```python
from build123d import *

# Parameters (mm, degrees)
SKETCH1_R           = 6
BOSS_EXTRUDE1_DEPTH = 44
SKETCH2_W           = 88
SKETCH2_H           = 20
CUT_EXTRUDE1_DEPTH  = 159.811208672
FILLET1_R           = 5


with BuildPart() as part:
    # Sketch1 → Boss-Extrude1 (new body)
    with BuildSketch(Plane.XY):
        with BuildLine():
            Line((0, 11), (140, 11))
            ThreePointArc((140, 11), (151, 0), (140, -11))
            Line((140, -11), (0, -11))
            ThreePointArc((0, -11), (-11, 0), (0, 11))
        make_face()
        Circle(SKETCH1_R, mode=Mode.SUBTRACT)
        with Locations((140, 0)):
            Circle(SKETCH1_R, mode=Mode.SUBTRACT)
    extrude(amount=BOSS_EXTRUDE1_DEPTH)

    # Sketch2 → Cut-Extrude1 (cut, through all)
    with BuildSketch(Plane(origin=(0, 11, 0), x_dir=(1, 0, 0), z_dir=(0, 1, 0))):
        with Locations((-11, -22)):
            Rectangle(SKETCH2_W, SKETCH2_H)
    extrude(amount=-CUT_EXTRUDE1_DEPTH, mode=Mode.SUBTRACT)

    # Fillet1
    fillet1_edges = [part.edges().sort_by_distance(p)[0] for p in [
        (33, 0, 32),
        (33, 0, 12),
    ]]
    fillet(fillet1_edges, radius=FILLET1_R)


solid = part.part
```
Check sheet for the modelled part. Datum: model origin and axes. Units: mm. A direction names the side the tool comes from. Give positions to 0.01 mm unless a question says otherwise; leave off trailing zeros. Order: outer loops, then holes, each group sorted by start corner. A loop starts at its lowest first (then second) coordinate and runs counter-clockwise, first axis right, second up. Notation, with made-up numbers: M 9,30 L 18,30 A21 cw 18,47 Z; hole C -13.5,-17 d3. An arc over 180 degrees is marked long. Answer in a Markdown table with one row per item.
1) Cross-section at D-D, the plane y = -9. Enter the section's corners in (x, z), plus the area to 3 significant figures.
Filled sheet:
| item | result |
|---|---|
| outline | M -6.32,0 L 146.32,0 L 146.32,44 L -6.32,44 L -6.32,32 L 28,32 A5 cw 33,27 L 33,17 A5 cw 28,12 L -6.32,12 Z |
| area | 5,940 mm2 |
2) Cross-section at C-C, the plane z = 8. Enter the section's corners in (x, y).
Filled sheet:
| item | result |
|---|---|
| outline | M 0,-11 L 140,-11 A11 ccw 140,11 L 0,11 A11 ccw Z; hole C 0,0 d12; hole C 140,0 d12 |
3) Cross-section at B-B, the plane x = 10. Enter the section's corners in (y, z), plus the area to 3 significant figures.
Filled sheet:
| item | result |
|---|---|
| outline | M -11,0 L 11,0 L 11,12 L -11,12 Z; M -11,32 L 11,32 L 11,44 L -11,44 Z |
| area | 528 mm2 |
4) Thickness scan on L1, parallel to X at y = 2, z = 6; L2, parallel to Y at x = 140, z = 10; L3, parallel to X at y = 5, z = 37.5. Record the ranges inside material, lowest first. Write a range as [from, to].
Filled sheet:
| item | result |
|---|---|
| L1 | x = [-10.82, -5.66], [5.66, 134.34], [145.66, 150.82] |
| L2 | y = [-11, -6], [6, 11] |
| L3 | x = [-9.8, -3.32], [3.32, 136.68], [143.32, 149.8] |
5) Release check for a two-part mould opening along Y. For faces 3 (the cylindrical face through (-6, 0, 6)), 4 (the cylindrical face through (-6, 0, 38)), 5 (the cylindrical face through (-11, 0, 38)), 6 (the flat face through (71, 0, 44)) record: +Y half, -Y half, draft (parallel to the pull), parting line (faces both ways), or undercut.
Filled sheet:
| item | result |
|---|---|
| face 3 | undercut |
| face 4 | undercut |
| face 5 | parting line |
| face 6 | draft |
6) Cross-section at A-A, the plane y = 0. Enter the section's corners in (x, z), plus the area to 3 significant figures.
Filled sheet:
| item | result |
|---|---|
| outline | M -11,0 L -6,0 L -6,12 L -11,12 Z; M -11,32 L -6,32 L -6,44 L -11,44 Z; M 6,0 L 134,0 L 134,44 L 6,44 L 6,32 L 28,32 A5 cw 33,27 L 33,17 A5 cw 28,12 L 6,12 Z; M 146,0 L 151,0 L 151,44 L 146,44 Z |
| area | 5,440 mm2 |
7) Access from +Z, -Z, +X, -X, +Y, -Y to the whole of each face (thin tool, end or side, straight path). Record for faces 1 (the cylindrical face through (31, 0, 31)), 2 (the flat face through (69, 11, 22)).
Filled sheet:
| item | result |
|---|---|
| face 1 | -X, +Y, -Y |
| face 2 | +Z, -Z, +X, -X, +Y |
8) Gauge pin test, flat ends, axial feed: P1, Ø3, axis at y = -2.5, z = 22.5, coming from the -X side; P2, Ø1.5, axis at y = -1, z = 38.5, coming from the -X side. Record the tip position at first contact, or that the pin passes through.
Filled sheet:
| item | result |
|---|---|
| P1 | stops at x = 33 |
| P2 | stops at x = -11 |
